Geometry: final body of the model. Coordinates: model frame, mm. A direction names the side the tool comes from. Coordinates: 2 decimals unless noted, no trailing zeros. Order: outer loops, then holes, each group sorted by start corner. A loop starts at its lowest first (then second) coordinate and runs counter-clockwise, first axis right, second up. Notation, with made-up numbers: (-10.5, 35) - (44.5, 35) arc R16 cw to (44.5, 60) - close; hole circle Ø3 at (36, -0.75). An arc over 180 degrees is marked (long way). Use a Markdown table: item, result. Add a question column.
```python
from build123d import *

# Parameters (mm, degrees)
BOSS_EXTRUDE1_DEPTH = 10.9474
CUT_EXTRUDE1_DEPTH  = 66.230102934
CUT_EXTRUDE2_DEPTH  = 63.46692107
SKETCH4_W           = 29.0576
SKETCH4_H           = 2.9464
CUT_EXTRUDE3_DEPTH  = 10.9474
CUT_EXTRUDE4_DEPTH  = 6.5278
FILLET1_R           = 4.0005
CUT_EXTRUDE5_DEPTH  = 66.230102934
CUT_EXTRUDE6_DEPTH  = 4.0005
CUT_EXTRUDE7_DEPTH  = 4.0005
SKETCH9_R           = 2.8321
CUT_EXTRUDE8_DEPTH  = 63.46692107
SKETCH10_R          = 3.2639
CUT_EXTRUDE9_DEPTH  = 1.143
CUT_EXTRUDE10_START = -1.143
SKETCH11_R          = 3.2639
CUT_EXTRUDE10_DEPTH = 1.143
CUT_EXTRUDE11_DEPTH = 2.9972
CUT_EXTRUDE13_START = -2.9972
CUT_EXTRUDE13_DEPTH = 2.9972
SKETCH14_R          = 1.27
CUT_EXTRUDE14_DEPTH = 63.46692107
SKETCH15_R          = 0.8382
BOSS_EXTRUDE2_DEPTH = 2.9972
CUT_EXTRUDE15_DEPTH = 4.0005
CUT_EXTRUDE16_DEPTH = 4.0005
SCALE1_SCALE        = 0.6


with BuildPart() as part:
    # Sketch1 → Boss-Extrude1 (new body)
    with BuildSketch(Plane(origin=(0, 0, 0), x_dir=(1, 0, 0), z_dir=(0, 1, 0))):
        with BuildLine():
            Line((0, 11.5316), (0, -11.5316))
            ThreePointArc((0, -11.5316), (-0.877859555, -13.650940445), (-2.9972, -14.5288))
            Line((-2.9972, -14.5288), (-3.683, -14.5288))
            Line((-3.683, -14.5288), (-3.683, -23.0505))
            Line((-3.683, -23.0505), (2.921, -23.0505))
            Line((2.921, -23.0505), (2.921, -19.05))
            Line((2.921, -19.05), (44.831, -19.05))
            Line((44.831, -19.05), (44.831, -14.5415))
            Line((44.831, -14.5415), (9.017, -14.5415))
            ThreePointArc((9.017, -14.5415), (6.897659555, -13.663640445), (6.0198, -11.5443))
            Line((6.0198, -11.5443), (6.0198, 11.5443))
            ThreePointArc((6.0198, 11.5443), (6.897659555, 13.663640445), (9.017, 14.5415))
            Line((9.017, 14.5415), (44.831, 14.5415))
            Line((44.831, 14.5415), (44.831, 19.05))
            Line((44.831, 19.05), (2.921, 19.05))
            Line((2.921, 19.05), (2.921, 23.0505))
            Line((2.921, 23.0505), (-3.683, 23.0505))
            Line((-3.683, 23.0505), (-3.683, 14.5288))
            Line((-3.683, 14.5288), (-2.9972, 14.5288))
            ThreePointArc((-2.9972, 14.5288), (-0.877859555, 13.650940445), (0, 11.5316))
        make_face()
    extrude(amount=BOSS_EXTRUDE1_DEPTH)

    # Sketch2 → Cut-Extrude1 (cut, through all)
    with BuildSketch(Plane.XY.offset(23.0505)):
        Polygon((-0.17535838, 0), (-3.683, 5.6134), (-3.683, 0), align=None)
    extrude(amount=-CUT_EXTRUDE1_DEPTH, mode=Mode.SUBTRACT)

    # Sketch3 → Cut-Extrude2 (cut, through all)
    with BuildSketch(Plane.XY.offset(19.05)):
        with BuildLine():
            Line((4.572, 8.001), (44.831, 8.001))
            Line((44.831, 8.001), (44.831, 10.9474))
            Line((44.831, 10.9474), (2.921, 10.9474))
            Line((2.921, 10.9474), (2.921, 9.652))
            ThreePointArc((2.921, 9.652), (3.404566704, 8.484566704), (4.572, 8.001))
        make_face()
    extrude(amount=-CUT_EXTRUDE2_DEPTH, mode=Mode.SUBTRACT)

    # Sketch4 → Cut-Extrude3 (cut)
    with BuildSketch(Plane(origin=(6.0198, 0, 0), x_dir=(0, 0, -1), z_dir=(1, 0, 0))):
        with Locations((0, 9.4742)):
            Rectangle(SKETCH4_W, SKETCH4_H)
    extrude(amount=-CUT_EXTRUDE3_DEPTH, mode=Mode.SUBTRACT)

    # Sketch5 → Cut-Extrude4 (cut)
    with BuildSketch(Plane(origin=(0, 8.001, 0), x_dir=(1, 0, 0), z_dir=(0, 1, 0))):
        with BuildLine():
            Line((0.9398, -12.446), (0.9398, 12.446))
            ThreePointArc((0.9398, 12.446), (3.0099, 14.5161), (5.08, 12.446))
            Line((5.08, 12.446), (5.08, -12.446))
            ThreePointArc((5.08, -12.446), (3.0099, -14.5161), (0.9398, -12.446))
        make_face()
    extrude(amount=-CUT_EXTRUDE4_DEPTH, mode=Mode.SUBTRACT)

    # Fillet1
    fillet1_edges = [part.edges().sort_by_distance(p)[0] for p in [
        (44.831, 8.001, -16.79575),
        (44.831, 0, -16.79575),
        (44.831, 0, 16.79575),
        (44.831, 8.001, 16.79575),
    ]]
    fillet(fillet1_edges, radius=FILLET1_R - 0.0001)  # a hair under: the kernel refuses the full size

    # Sketch6 → Cut-Extrude5 (cut, through all)
    with BuildSketch(Plane.XY.offset(23.0505)):
        Polygon((-3.683, 10.9474), (2.921, 9.782936619), (2.921, 10.9474), align=None)
    extrude(amount=-CUT_EXTRUDE5_DEPTH, mode=Mode.SUBTRACT)

    # Sketch7 → Cut-Extrude6 (cut)
    with BuildSketch(Plane.XY.offset(23.0505)):
        Polygon((-3.683, 8.987220468), (-3.683, 5.6134), (-0.17535838, 0), (2.921, 0), (2.921, 7.822757088), align=None)
    extrude(amount=-CUT_EXTRUDE6_DEPTH, mode=Mode.SUBTRACT)

    # Sketch8 → Cut-Extrude7 (cut)
    with BuildSketch(Plane(origin=(0, 0, -23.0505), x_dir=(-1, 0, 0), z_dir=(0, 0, -1))):
        Polygon((3.683, 8.987220468), (-2.921, 7.822757088), (-2.921, 0), (0.17535838, 0), (3.683, 5.6134), align=None)
    extrude(amount=-CUT_EXTRUDE7_DEPTH, mode=Mode.SUBTRACT)

    # Sketch9 → Cut-Extrude8 (cut, through all)
    with BuildSketch(Plane(origin=(0, 0, -19.05), x_dir=(-1, 0, 0), z_dir=(0, 0, -1))):
        with Locations((-40.8305, 4.0005)):
            Circle(SKETCH9_R)
    extrude(amount=-CUT_EXTRUDE8_DEPTH, mode=Mode.SUBTRACT)

    # Sketch10 → Cut-Extrude9 (cut)
    with BuildSketch(Plane(origin=(0, 0, -19.05), x_dir=(-1, 0, 0), z_dir=(0, 0, -1))):
        with Locations((-40.8305, 4.0005)):
            Circle(SKETCH10_R)
    extrude(amount=-CUT_EXTRUDE9_DEPTH, mode=Mode.SUBTRACT)

    # Sketch11 → Cut-Extrude10 (cut)
    with BuildSketch(Plane.XY.offset(19.05).offset(CUT_EXTRUDE10_START)):
        with Locations(Location((40.8305, 4.0005, 0), (0, 0, 180))):
            Circle(SKETCH11_R)
    extrude(amount=CUT_EXTRUDE10_DEPTH, mode=Mode.SUBTRACT)

    # Sketch12 → Cut-Extrude11 (cut)
    with BuildSketch(Plane.XY.offset(19.05)):
        with BuildLine():
            Line((33.655, 1.4605), (10.795, 1.4605))
            ThreePointArc((10.795, 1.4605), (8.255, 4.0005), (10.795, 6.5405))
            Line((10.795, 6.5405), (33.655, 6.5405))
            ThreePointArc((33.655, 6.5405), (36.195, 4.0005), (33.655, 1.4605))
        make_face()
    extrude(amount=-CUT_EXTRUDE11_DEPTH, mode=Mode.SUBTRACT)

    # Sketch13 → Cut-Extrude13 (cut)
    with BuildSketch(Plane(origin=(0, 0, -19.05), x_dir=(-1, 0, 0), z_dir=(0, 0, -1)).offset(CUT_EXTRUDE13_START)):
        with BuildLine():
            Line((-33.655, 6.5405), (-10.795, 6.5405))
            ThreePointArc((-10.795, 6.5405), (-8.255, 4.0005), (-10.795, 1.4605))
            Line((-10.795, 1.4605), (-33.655, 1.4605))
            ThreePointArc((-33.655, 1.4605), (-36.195, 4.0005), (-33.655, 6.5405))
        make_face()
    extrude(amount=CUT_EXTRUDE13_DEPTH, mode=Mode.SUBTRACT)

    # Sketch14 → Cut-Extrude14 (cut, through all)
    with BuildSketch(Plane(origin=(0, 0, -19.05), x_dir=(-1, 0, 0), z_dir=(0, 0, -1))):
        with Locations((-3.0099, 4.0005)):
            Circle(SKETCH14_R)
    extrude(amount=-CUT_EXTRUDE14_DEPTH, mode=Mode.SUBTRACT)

    # Sketch15 → Boss-Extrude2 (add)
    with BuildSketch(Plane.XZ):
        with BuildLine():
            Line((-5.1816, -2.54), (-5.1816, 2.54))
            Line((-5.1816, 2.54), (-2.499999953, 2.54))
            ThreePointArc((-2.499999953, 2.54), (-0.732233033, 3.272233033), (0, 5.039999953))
            Line((0, 5.039999953), (0, -5.039999953))
            ThreePointArc((0, -5.039999953), (-0.732233033, -3.272233033), (-2.499999953, -2.54))
            Line((-2.499999953, -2.54), (-5.1816, -2.54))
        make_face()
        with Locations(Location((-3.657652297, 0, 0), (0, 0, 270))):
            Circle(SKETCH15_R, mode=Mode.SUBTRACT)
    extrude(amount=-BOSS_EXTRUDE2_DEPTH)

    # Sketch16 → Cut-Extrude15 (cut)
    with BuildSketch(Plane.XY.offset(19.05)):
        Polygon((2.921, 7.822757088), (-3.683, 8.987220468), (-3.683, 9.24285301), (2.921, 8.078389629), align=None)
    extrude(amount=CUT_EXTRUDE15_DEPTH, mode=Mode.SUBTRACT)

    # Sketch17 → Cut-Extrude16 (cut)
    with BuildSketch(Plane(origin=(0, 0, -19.05), x_dir=(-1, 0, 0), z_dir=(0, 0, -1))):
        Polygon((-2.921, 8.078389629), (3.683, 9.24285301), (3.683, 8.987220468), (-2.921, 7.822757088), align=None)
    extrude(amount=CUT_EXTRUDE16_DEPTH, mode=Mode.SUBTRACT)


with BuildPart() as part_1:
    # Scale1: scaled about (13.203263525, 4.213395444, -2.977e-06)
    add(part.part.scale(SCALE1_SCALE).moved(Location((5.28130541, 1.685358178, -1.191e-06))))


solid = part_1.part
```
1) Set-up query: faces 1 (the face through (4, 3.484, 0)), 2 (the face through (19, 5.61, 11)), 3 (the face through (7, 2.569, 0)), 4 (the face through (3, 3, -1.524)). Return all of +Z, -Z, +X, -X, +Y, -Y with unobstructed straight access to the full face (end or side cutting, diameter ignored); none if empty.
2) Ray query, line 1 along Z through (x, y) = (26, 3); line 2 along X through (y, z) = (5.25, -11) (1 decimal); line 3 along Z through (x, y) = (11, 2.25). Return the intervals inside material, ascending.
3) Section B-B (z = 3.5). Return loops of the section in (x, y).
4) Draft query along X for faces 5 (the face through (3.072, 7, 11)), 6 (the face through (6.688, 4.99, 8.644)), 7 (the face through (31.46, 5.8, 10.06)). Return one class per face: pulls with the +X half, pulls with the -X half, needs draft (parallel to the pull), parting line crosses it, or undercut.
5) Pin query (flat end, axial travel): pin 1 (1.8 mm diameter, centred on x = 7.09, y = 4.09, fed in from +Z); pin 2 (1 mm diameter, centred on y = 2.5, z = 7.5, fed in from -X); pin 3 (1.2 mm diameter, centred on x = 7, z = -3, fed in from +Y). Return the tip coordinate at first contact, or that it passes through.
6) Section A-A (x = 23). Return loops of the section in (y, z).
Values follow:
| question | item | result |
|---|---|---|
| 1 | face 1 | -X, +Y |
| 1 | face 2 | +Z |
| 1 | face 3 | +Y |
| 1 | face 4 | -Z, -X, +Y, -Y |
| 2 | line 1 | z = -9.63 to -8.72, 8.72 to 9.63 |
| 2 | line 2 | x = 3.1 to 10.8, 26.5 to 28.2, 31.4 to 31.9 |
| 2 | line 3 | z = -11.43 to -8.72, 8.72 to 11.43 |
| 3 | outline | (5.28, 1.69) - (8.89, 1.69) - (8.89, 6.49) - (8.33, 6.49) - (8.33, 2.57) - (5.85, 2.57) - (5.85, 6.49) - (5.28, 6.49) - close |
| 4 | face 5 | pulls with the -X half |
| 4 | face 6 | undercut |
| 4 | face 7 | pulls with the +X half |
| 5 | pin 1 | stops at z = 11.43 |
| 5 | pin 2 | stops at x = 4.92 |
| 5 | pin 3 | stops at y = 2.57 |
| 6 | outline | (1.69, -11.43) - (2.56, -11.43) - (2.56, -9.63) - (5.61, -9.63) - (5.61, -11.43) - (6.49, -11.43) - (6.49, -8.72) - (1.69, -8.72) - close; (1.69, 8.72) - (6.49, 8.72) - (6.49, 11.43) - (5.61, 11.43) - (5.61, 9.63) - (2.56, 9.63) - (2.56, 11.43) - (1.69, 11.43) - close |
